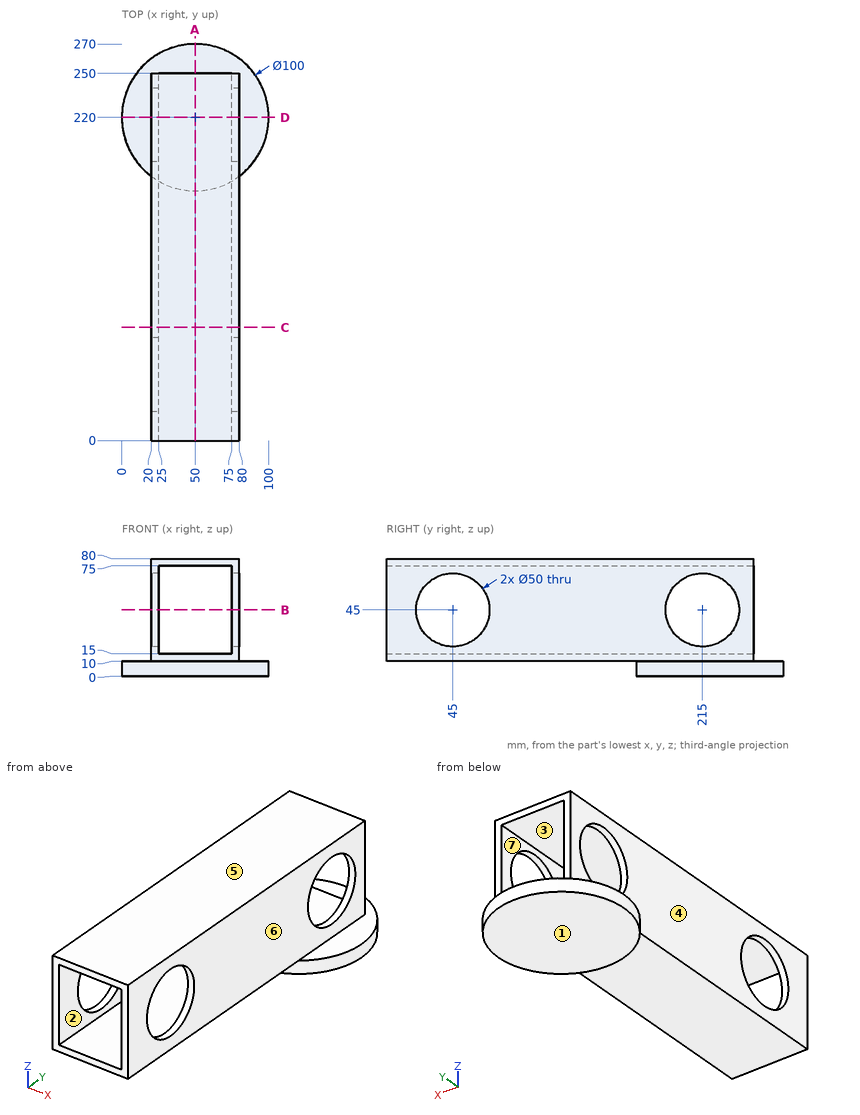
Print and shaded views of the part. All mm, measured from the part's lowest x, y and z. A direction names the side the tool comes from. Coordinates: 2 decimals unless noted, no trailing zeros. Order: outer loops, then holes, each group sorted by start corner. A loop starts at its lowest first (then second) coordinate and runs counter-clockwise, first axis right, second up. Notation, with made-up numbers: (-14.5, -29) - (-5.5, -29) arc R17 ccw to (-5.5, -13) - close; hole circle Ø11 at (-23, -21.75). An arc over 180 degrees is marked (long way). Return JSON: item names as keys, results as strings. Group by question number.
Item 1: Pull direction X, two halves, no side cores. Call the marked faces 1, 2, 3 and 4: pulls with the +X half, pulls with the -X half, needs draft (parallel to the pull), parting line crosses it, or undercut.
Item 2: Pin check, flat tips, straight feed: pin 1 (5 mm diameter, centred on y = 90, z = 19, fed in from -X); pin 2 (25 mm diameter, centred on x = 61, y = 166, fed in from -Z); pin 3 (18 mm diameter, centred on x = 57.5, y = 73, fed in from -Z); pin 4 (10 mm diameter, centred on y = 208.5, z = 15.5, fed in from +X). Stop position of each tip, or through.
Item 3: Drill centre lines: probe 1 along X at (y, z) = (121.5, 39); probe 2 along Z at (x, y) = (76.75, 45); probe 3 along Z at (x, y) = (63.5, 152.5). Where is each one in solid material? Low to high. Write a range as from..to.
Item 4: Cut at B-B (z = 45). List the corners of the cut face in (x, y).
Item 5: Cut at D-D (y = 220). List the corners of the cut face in (x, z).
Item 6: Cut at A-A (x = 50). List the corners of the cut face in (y, z).
Item 7: Which spindle directions (+Z, -Z, +X, -X, +Y, -Y) get a long thin tool onto all of the face, cutting with end or side? Do the marked faces 5, 6 and 7. Say none if no direction does.
Item 8: Cut at C-C (y = 77). List the corners of the cut face in (x, z), plus the area to 3 significant figures.
Check values:
{
 "1": {"face 1": "needs draft", "face 2": "undercut", "face 3": "undercut", "face 4": "pulls with the -X half"},
 "2": {"pin 1": "stops at x = 20", "pin 2": "stops at z = 0", "pin 3": "stops at z = 10", "pin 4": "stops at x = 80"},
 "3": {"probe 1": "x = 20..25, 75..80", "probe 2": "z = 10..20, 70..80", "probe 3": "z = 10..15, 75..80"},
 "4": {"outline": "(20, 0) - (25, 0) - (25, 20) - (20, 20) - close; (20, 70) - (25, 70) - (25, 190) - (20, 190) - close; (20, 240) - (25, 240) - (25, 250) - (20, 250) - close; (75, 0) - (80, 0) - (80, 20) - (75, 20) - close; (75, 70) - (80, 70) - (80, 190) - (75, 190) - close; (75, 240) - (80, 240) - (80, 250) - (75, 250) - close"},
 "5": {"outline": "(0, 0) - (100, 0) - (100, 10) - (80, 10) - (80, 20.51) - (75, 20.51) - (75, 15) - (25, 15) - (25, 20.51) - (20, 20.51) - (20, 10) - (0, 10) - close; (20, 69.49) - (25, 69.49) - (25, 75) - (75, 75) - (75, 69.49) - (80, 69.49) - (80, 80) - (20, 80) - close"},
 "6": {"outline": "(0, 10) - (170, 10) - (170, 0) - (270, 0) - (270, 10) - (250, 10) - (250, 15) - (0, 15) - close; (0, 75) - (250, 75) - (250, 80) - (0, 80) - close"},
 "7": {"face 5": "+Z, +X, -X, +Y, -Y", "face 6": "+Z, +X, +Y, -Y", "face 7": "+Y, -Y"},
 "8": {"outline": "(20, 10) - (80, 10) - (80, 80) - (20, 80) - close; hole (25, 15) - (75, 15) - (75, 75) - (25, 75) - close", "area": "1,200 mm2"}
}
